Autodesk Inventor part; units mm, degrees
ref_plane "YZ Plane" through (0, 0, 0) normal (1, 0, 0) x (0, 1, 0)
ref_plane "XZ Plane" through (0, 0, 0) normal (0, 1, 0) x (-1, 0, 0)
ref_plane "XY Plane" through (0, 0, 0) normal (0, 0, 1) x (1, 0, 0)
sketch "草圖1" plane through (0, 0, 0) normal (0, 1, 0) x (-1, 0, 0)
  line L0 (24.1962, 30) -> (-19.5, 30)
  line L1 (-22.5, 27) -> (-22.5, -27)
  line L2 (-22.5, -30) -> (24.1827, -30)
  line L3 (25, 30) -> (17.3, 30)
  line L4 (25.6962, 29.5981) -> (33.7194, 24.9658)
  line L5 (-19.5, -30) -> (26.7, -30)
  line L6 (27.1371, -27.5209) -> (35.6587, 20.8071)
  line L7 (-14.8, -27) -> (-8.8, -27)
  line L8 (-8.8, -27) -> (-8.8, -24)
  line L9 (-8.8, -24) -> (-14.8, -24)
  line L10 (-14.8, -24) -> (-14.8, -27)
  line L11 (-14.8, -22.5) -> (-11.8, -22.5)
  line L12 (-11.8, -22.5) -> (-11.8, -12.5)
  line L13 (-11.8, -12.5) -> (-14.8, -12.5)
  line L14 (-14.8, -12.5) -> (-14.8, -22.5)
  line L15 (-11.8, -12.5) -> (-13.3, -12.5)
  circle A0 centre (-13.3, 0) radius 1.5
  line L16 (-11.8, 22.5) -> (-14.8, 22.5)
  line L17 (-14.8, 22.5) -> (-14.8, 12.5)
  line L18 (-14.8, 12.5) -> (-11.8, 12.5)
  line L19 (-11.8, 12.5) -> (-11.8, 22.5)
  circle A1 centre (-5.3, -25.5) radius 1.5
  line L20 (4.2, -24) -> (-1.8, -24)
  line L21 (-1.8, -24) -> (-1.8, -27)
  line L22 (-1.8, -27) -> (4.2, -27)
  line L23 (4.2, -27) -> (4.2, -24)
  line L24 (9.2, -21) -> (21.2, -21)
  line L25 (21.2, -21) -> (21.2, 2)
  line L26 (21.2, 2) -> (9.2, 2)
  line L27 (9.2, 2) -> (9.2, -21)
  line L28 (9.2, -21) -> (9.2, -9.5)
  circle A2 centre (6.2, -9.5) radius 1.5
  circle A3 centre (24.2, -9.5) radius 1.5
  line L29 (5, 19.8) -> (15, 19.8)
  line L30 (15, 19.8) -> (15, 22.8)
  line L31 (15, 22.8) -> (5, 22.8)
  line L32 (5, 22.8) -> (5, 19.8)
  line L33 (-22.5, -30) -> (-22.5, -27)
  line L34 (-22.5, -27) -> (-14.8, -27)
  line L35 (-3.8, 12.5) -> (-9.8, 12.5)
  line L36 (-9.8, 12.5) -> (-9.8, 2.5)
  line L37 (-9.8, 2.5) -> (-3.8, 2.5)
  line L38 (-3.8, 2.5) -> (-3.8, 12.5)
  line L39 (15, 22.8) -> (15, 21.3)
  line L40 (15, 21.3) -> (29.9, 21.3)
  circle A4 centre (29.9, 21.3) radius 1.5
  arc A5 (25.6962, 29.5981) -> (24.1962, 30) centre (24.1962, 27) ccw
  arc A6 (35.6587, 20.8071) -> (33.7194, 24.9658) centre (31.7194, 21.5017) ccw
  arc A7 (24.1827, -30) -> (27.1371, -27.5209) centre (24.1827, -27) ccw
  arc A8 (-22.5, -27) -> (-19.5, -30) centre (-19.5, -27) ccw
  arc A9 (-19.5, 30) -> (-22.5, 27) centre (-19.5, 27) ccw
  point P0 (-22.5, 30)
  point P1 (25, -30)
  dimension "d0" = 60
  dimension "d1" = 47.5
  dimension "d43" = 49.2
  dimension "d44" = 110
  dimension "d46" = 3
  dimension "d47" = 1.5
  dimension "d48" = 3
  dimension "d49" = 10
  dimension "d50" = 3
  dimension "d51" = 1.5
  dimension "d53" = 3
  dimension "d54" = 3
  dimension "d55" = 10
  dimension "d56" = 3
  dimension "d61" = 3
  dimension "d62" = 6
  dimension "d63" = 3
  dimension "d67" = 12
  dimension "d68" = 23
  dimension "d69" = 11.5
  dimension "d72" = 3
  dimension "d73" = 3
  dimension "d74" = 10
  dimension "d75" = 3
  dimension "d76" = 3
  dimension "d77" = 7.7
  dimension "d78" = 6
  dimension "d79" = 10
  dimension "d80" = 32.5
  dimension "d81" = 12.7
  dimension "d82" = 14.9
  dimension "d83" = 3
  dimension "d84" = 3
  dimension "d85" = 4
extrude "擠出2" add sketch "草圖1" along normal mid plane 3
properties part number "板子2"
Can you work these out from the model? Positions are in its coordinate system, mm. A direction names the side the tool comes from. Coordinates: 2 decimals unless noted, no trailing zeros. Loops run counter-clockwise (first coordinate to the right, second up) from the corner with the lowest first, then second, coordinate; pieces in that order, holes last.
1) I need wall thicknesses on probe 1 along Z at (x, y) = (13.3, 0.05); probe 2 along X at (y, z) = (0.7, 21.3); probe 3 along Z at (x, y) = (5.3, -0.25). Which ranges of each line are inside material? Lowest first, please.
2) Imagine slicing it at C-C on z = -18. List the corners of the cut face in (x, y) for me, plus the area to 3 significant figures.
3) Imagine slicing it at D-D on x = -1.5. List the corners of the cut face in (y, z) for me, plus the area to 3 significant figures.
4) Imagine slicing it at B-B on z = -5.5. List the corners of the cut face in (x, y) for me.
5) For pin 1 (2.5 mm diameter, centred on x = -6.2, z = -9.5, fed in from -Y); pin 2 (1.5 mm diameter, centred on y = 0.5, z = 7.5, fed in from -X), each with a flat end and sliding along its axis, tell me the tip position at first contact or that it passes through.
6) Thinking about a two-plate mould opening in Z: for faces 1 (the flat face through (-1, 0, -30)), 2 (the flat face through (-6, -1.5, 0)), 3 (the flat face through (11.8, 0, 17)), which applies, pulls with the +Z half, pulls with the -Z half, needs draft (parallel to the pull), parting line crosses it, or undercut?
7) Imagine slicing it at A-A on x = -11. List the corners of the cut face in (y, z) for me.
8) Which directions (+Z, -Z, +X, -X, +Y, -Y) give clear straight access to the entire face, cutting with the end or side of a thin tool? Please do faces 4 (the flat face through (22.5, 0, -1)), 5 (the flat face through (13, 0, -22.5)).
Completed:
1. probe 1: z = -30 to -27, -24 to -22.5, -12.5 to -1.5, 1.5 to 12.5, 22.5 to 30
1. probe 2: x = -35.71 to -31.4, -28.4 to -15, -5 to 11.8, 14.8 to 22.5
1. probe 3: z = -30 to -27, -24 to 2.5, 12.5 to 30
2. outline: (-28.82, -1.5) - (-21.2, -1.5) - (-21.2, 1.5) - (-28.82, 1.5) - close; (-9.2, -1.5) - (11.8, -1.5) - (11.8, 1.5) - (-9.2, 1.5) - close; (14.8, -1.5) - (22.5, -1.5) - (22.5, 1.5) - (14.8, 1.5) - close
2. area: 109 mm2
3. outline: (-1.5, -30) - (1.5, -30) - (1.5, -27) - (-1.5, -27) - close; (-1.5, -24) - (1.5, -24) - (1.5, 30) - (-1.5, 30) - close
3. area: 171 mm2
4. outline: (-31.02, -1.5) - (-21.2, -1.5) - (-21.2, 1.5) - (-31.02, 1.5) - close; (-9.2, -1.5) - (22.5, -1.5) - (22.5, 1.5) - (-9.2, 1.5) - close
5. pin 1: passes through
5. pin 2: stops at x = -33.44
6. face 1: pulls with the -Z half
6. face 2: needs draft
6. face 3: undercut
7. outline: (-1.5, -30) - (1.5, -30) - (1.5, -21) - (-1.5, -21) - close; (-1.5, 2) - (1.5, 2) - (1.5, 19.8) - (-1.5, 19.8) - close; (-1.5, 22.8) - (1.5, 22.8) - (1.5, 30) - (-1.5, 30) - close
8. face 4: +Z, -Z, +X, +Y, -Y
8. face 5: +Y, -Y
